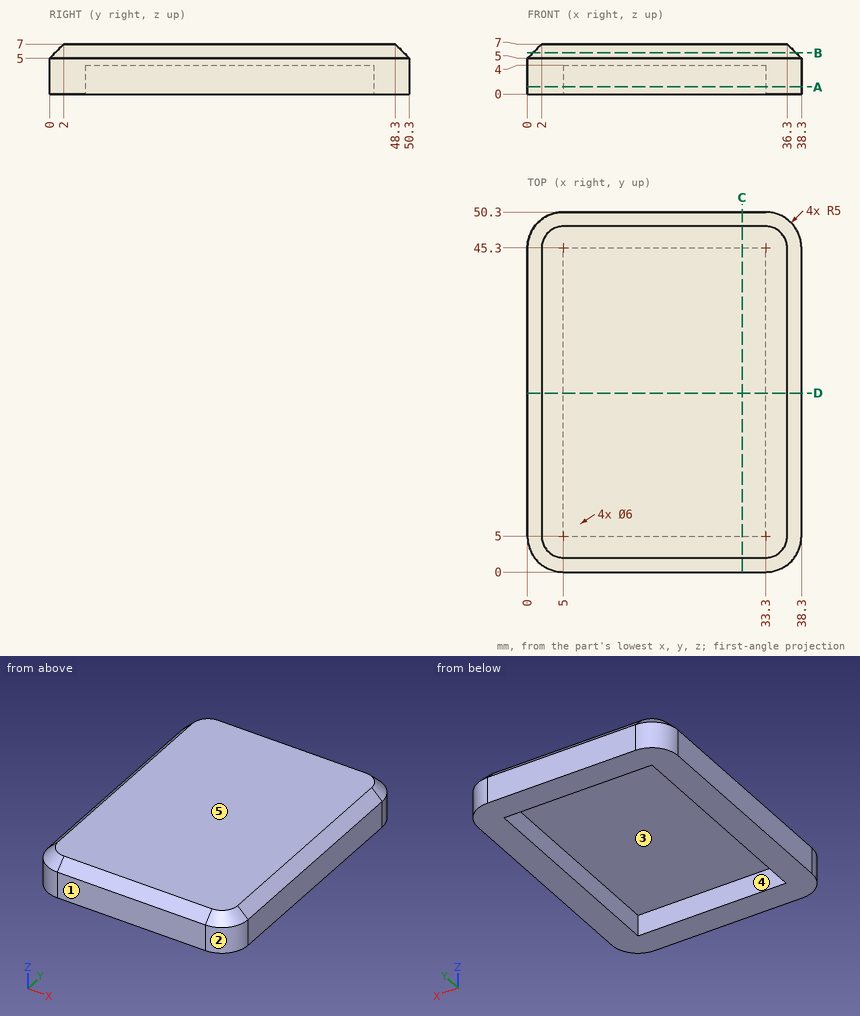
Job drawing, mm, ordinate dimensions from the low corner. One solid piece. A direction names the side the tool comes from. Coordinates: 2 decimals unless noted, no trailing zeros. Order: outer loops, then holes, each group sorted by start corner. A loop starts at its lowest first (then second) coordinate and runs counter-clockwise, first axis right, second up. Notation, with made-up numbers: (84, 49) - (123, 49) arc R26 cw to (123, 85) - close; hole circle Ø1 at (-4.5, 84). An arc over 180 degrees is marked (long way). Return JSON: item names as keys, results as strings. Group by question number.
1) Tool access for the marked faces 4 and 5: list every direction of +Z, -Z, +X, -X, +Y, -Y with a clear straight run to the whole face (end or side of a thin tool).
2) Saw through at D-D, the plane y = 25. Write the cut outline in (x, z).
3) Saw through at A-A, the plane z = 1. Write the cut outline in (x, y), plus the area to 3 significant figures.
4) Probe line 1 (Y direction, x = 17, z = 1.75); line 2 (X direction, y = 23, z = 3.5); line 3 (Z direction, x = 13.5, y = 43). List the from-to ranges inside material, lowest first. Write a range as from..to.
5) Mould opens along X. For the marked faces 1, 2 and 3 say: released by +X, released by -X, zero draft, split by the parting line, or undercut.
6) Flat gauge pin, fed straight in: P1, Ø1.5, axis at x = 18.5, y = 17.5, coming from the -Z side. Where does the tip first touch, or does it go through?
7) Saw through at C-C, the plane x = 30. Write the cut outline in (y, z), plus the area to 3 significant figures.
8) Saw through at B-B, the plane z = 5.75. Write the cut outline in (x, y).
Values found:
{
 "1": {"face 4": "-Z", "face 5": "+Z, +X, -X, +Y, -Y"},
 "2": {"outline": "(0, 0) - (5, 0) - (5, 4) - (33.3, 4) - (33.3, 0) - (38.3, 0) - (38.3, 5) - (36.3, 7) - (2, 7) - (0, 5) - close"},
 "3": {"outline": "(0, 5) arc R5 ccw to (5, 0) - (33.3, 0) arc R5 ccw to (38.3, 5) - (38.3, 45.3) arc R5 ccw to (33.3, 50.3) - (5, 50.3) arc R5 ccw to (0, 45.3) - close; hole (5, 5) - (33.3, 5) - (33.3, 45.3) - (5, 45.3) - close", "area": "765 mm²"},
 "4": {"line 1": "y = 0..5, 45.3..50.3", "line 2": "x = 0..5, 33.3..38.3", "line 3": "z = 4..7"},
 "5": {"face 1": "zero draft", "face 2": "released by +X", "face 3": "undercut"},
 "6": {"P1": "stops at z = 4"},
 "7": {"outline": "(0, 0) - (5, 0) - (5, 4) - (45.3, 4) - (45.3, 0) - (50.3, 0) - (50.3, 5) - (48.3, 7) - (2, 7) - (0, 5) - close", "area": "187 mm²"},
 "8": {"outline": "(0.75, 5) arc R4.25 ccw to (5, 0.75) - (33.3, 0.75) arc R4.25 ccw to (37.55, 5) - (37.55, 45.3) arc R4.25 ccw to (33.3, 49.55) - (5, 49.55) arc R4.25 ccw to (0.75, 45.3) - close"}
}
